Verification items for this drawing (mm, ordinates from the low corner). A direction names the side the tool comes from. Coordinates: 2 decimals unless noted, no trailing zeros. One line per item, written item: value. Start each with the question number.
1) Thickness scan on L1, parallel to Z at x = 15.5, y = 10 (1 decimal); L2, parallel to X at y = 35, z = 16.5; L3, parallel to Z at x = 13.5, y = 106.5. Record the ranges inside material, lowest first. Write a range as from..to.
2) Access from +Z, -Z, +X, -X, +Y, -Y to the whole of each face (thin tool, end or side, straight path). Record for the marked faces 1 and 2.
3) Go/stop test with flat-tipped pins: P1, Ø1, axis at x = 25, z = 20, coming from the -Y side; P2, Ø1, axis at y = 49.5, z = 14.5, coming from the -X side; P3, Ø5, axis at x = 26, y = 73, coming from the -Z side; P4, Ø1, axis at x = 13.5, y = 71, coming from the +Z side. Record where each tip stops, or that it passes through.
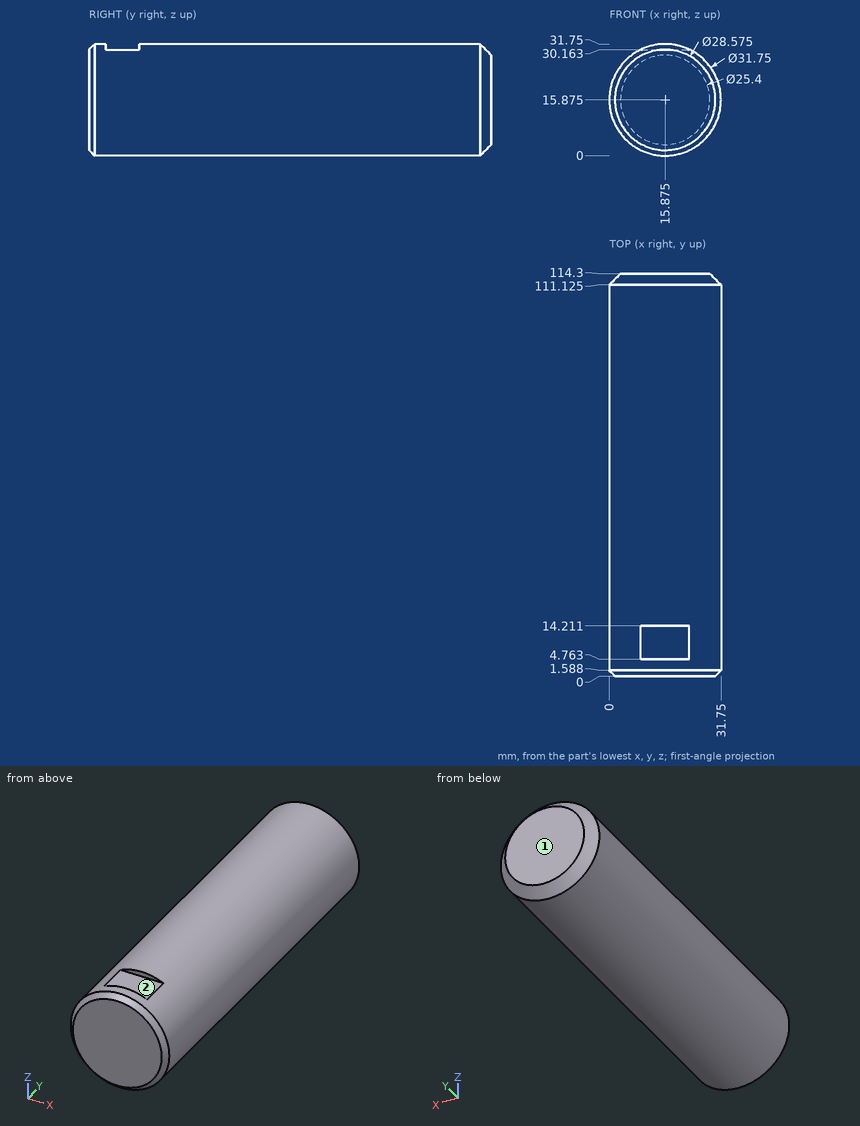
Final values:
1. L1: z = 0..30.2
1. L2: x = 0.01..31.74
1. L3: z = 0.18..31.57
2. face 1: +Z, -Z, +X, -X, +Y
2. face 2: +Z, +X, -X
3. P1: stops at y = 0
3. P2: stops at x = 0.02
3. P3: stops at z = 1.95
3. P4: stops at z = 31.64
